```python
from build123d import *

# Parameters (mm, degrees)
F1_DEPTH = 7.62
F2_SIZE  = 2.032


with BuildPart() as f1:
    # F0 (on Top) → F1 (new body)
    with BuildSketch(Plane.XY):
        Polygon((-4.650212, 0), (0, 0), (13.123814, 0), (27.571009, 15.396307), (32.54258, 15.396307), (44.767726, 15.396307), (44.767726, 0), (58.344088, 0), (61.602417, 0), (61.602417, 13.099327), (61.602417, 15.906334), (75.450297, 0), (77.894047, 0), (92.737518, 0), (67.757033, 31.506918), (92.737518, 59.383705), (78.075059, 59.383705), (75.39035, 59.383705), (61.602417, 43.997165), (61.602417, 59.383705), (58.344088, 59.383705), (47.120962, 59.383705), align=None)
        Polygon((44.043656, 38.960008), (48.304201, 38.960008), (52.189469, 38.960008), (52.189469, 25.352303), (36.440898, 25.352303), (32.180353, 25.352303), align=None, mode=Mode.SUBTRACT)
    extrude(amount=F1_DEPTH)

    # F2
    f2_edges = [f1.edges().sort_by_distance(p)[0] for p in [
        (21.235375, 29.691853, 7.62),
        (4.236801, 0, 7.62),
        (20.347412, 7.698154, 7.62),
        (36.169368, 15.396307, 7.62),
        (44.767726, 7.698154, 7.62),
        (53.185072, 0, 7.62),
        (61.602417, 7.953167, 7.62),
        (68.526357, 7.953167, 7.62),
        (84.093908, 0, 7.62),
        (80.247276, 15.753459, 7.62),
        (80.247276, 45.445312, 7.62),
        (84.063934, 59.383705, 7.62),
        (68.496384, 51.690435, 7.62),
        (61.602417, 51.690435, 7.62),
        (54.36169, 59.383705, 7.62),
        (38.112005, 32.156156, 7.62),
        (48.116563, 38.960008, 7.62),
        (52.189469, 32.156156, 7.62),
        (42.184911, 25.352303, 7.62),
        (21.235375, 29.691853, 0),
        (4.236801, 0, 0),
        (20.347412, 7.698154, 0),
        (36.169368, 15.396307, 0),
        (44.767726, 7.698154, 0),
        (53.185072, 0, 0),
        (61.602417, 7.953167, 0),
        (68.526357, 7.953167, 0),
        (84.093908, 0, 0),
        (80.247276, 15.753459, 0),
        (80.247276, 45.445312, 0),
        (84.063934, 59.383705, 0),
        (68.496384, 51.690435, 0),
        (61.602417, 51.690435, 0),
        (54.36169, 59.383705, 0),
        (38.112005, 32.156156, 0),
        (48.116563, 38.960008, 0),
        (52.189469, 32.156156, 0),
        (42.184911, 25.352303, 0),
    ]]
    chamfer(f2_edges, length=F2_SIZE)


solid = f1.part
```
Model file for the job. Use its own axes, mm. A direction names the side the tool comes from. Coordinates: 2 decimals unless noted, no trailing zeros. Loops run counter-clockwise (first coordinate to the right, second up) from the corner with the lowest first, then second, coordinate; pieces in that order, holes last. Notation, with made-up numbers: M -11.75,37 L -7.75,37 A18 ccw -7.75,63 Z; hole C -32,43.5 d1. An arc over 180 degrees is marked long. Use CSV: the item, a comma, the result in double quotes. Start each with the question number.
1. Band-saw the part on D-D, the plane y = 53. List the corners of the cut face in (x, z).
2. Probe probe 1 along X at (y, z) = (10.5, 4.25); probe 2 along X at (y, z) = (7.5, 2.75); probe 3 along X at (y, z) = (47, 1.25). List the from-to ranges inside material, lowest first. Write a range as [from, to].
3. Flat gauge pins, fed straight in: pin 1 (1.1 mm diameter, centred on y = 7.5, z = 3.5, fed in from -X); pin 2 (1.8 mm diameter, centred on x = 36, z = 4.5, fed in from -Y); pin 3 (4 mm diameter, centred on y = 50, z = 4, fed in from +X). Where does each tip first touch, or does it go through?
4. Tool access for faces 4 (the flat face through (41.15, 24.32, 6.62)), 5 (the flat face through (60.57, 10.52, 1)), 6 (the flat face through (67.4, 10.82, 6.62)): list every direction of +Z, -Z, +X, -X, +Y, -Y with a clear straight run to the whole face (end or side of a thin tool).
5. Band-saw the part on A-A, the plane z = 4.5. List the corners of the cut face in (x, y).
6. Two-plate mould, pull along X, no slides. Class faces 1 (the flat face through (83.97, 1.03, 1)), 2 (the flat face through (20.246, 7.59, 3.785)), 3 (the flat face through (22, 29, 1)): pulls with the +X half, pulls with the -X half, needs draft (parallel to the pull), parting line crosses it, or undercut.
7. Band-saw the part on B-B, the plane y = 11.5. List the corners of the cut face in (x, z).
8. Band-saw the part on C-C, the plane x = 82.5. List the corners of the cut face in (y, z), then the cut area to 3 significant figures.
Entries:
1,outline,"M 41.56,2.03 L 44.25,0 L 59.57,0 L 61.6,2.03 L 61.6,5.59 L 59.57,7.62 L 44.25,7.62 L 41.56,5.59 Z; M 69.67,2.03 L 72.4,0 L 84.29,0 L 87.02,2.03 L 87.02,5.59 L 84.29,7.62 L 72.4,7.62 L 69.67,5.59 Z"
2,probe 1,"x = [4.5, 22.98], [44.77, 61.6], [66.31, 84.41]"
2,probe 2,"x = [1.89, 20.16], [44.77, 61.6], [68.92, 86.79]"
2,probe 3,"x = [37.36, 60.82], [65.34, 80.59]"
3,pin 1,"stops at x = 1.41"
3,pin 2,"stops at y = 15.4"
3,pin 3,"stops at x = 86.12"
4,face 4,"+Z"
4,face 5,"-Z, -Y"
4,face 6,"+Z, -Y"
5,outline,"M -4.65,0 L 13.12,0 L 27.57,15.4 L 44.77,15.4 L 44.77,0 L 61.6,0 L 61.6,15.91 L 75.45,0 L 92.74,0 L 67.76,31.51 L 92.74,59.38 L 75.39,59.38 L 61.6,44 L 61.6,59.38 L 47.12,59.38 Z; hole M 32.18,25.35 L 52.19,25.35 L 52.19,38.96 L 44.04,38.96 Z"
6,face 1,"needs draft"
6,face 2,"undercut"
6,face 3,"pulls with the -X half"
7,outline,"M 5.38,2.03 L 8.07,0 L 21.13,0 L 23.91,2.03 L 23.91,5.59 L 21.13,7.62 L 8.07,7.62 L 5.38,5.59 Z; M 44.77,2.03 L 46.8,0 L 59.57,0 L 61.6,2.03 L 61.6,5.59 L 59.57,7.62 L 46.8,7.62 L 44.77,5.59 Z; M 65.44,2.03 L 68.13,0 L 81.03,0 L 83.62,2.03 L 83.62,5.59 L 81.03,7.62 L 68.13,7.62 L 65.44,5.59 Z"
8,outline,"M 0,2.03 L 2.03,0 L 9.64,0 L 12.91,2.03 L 12.91,5.59 L 9.64,7.62 L 2.03,7.62 L 0,5.59 Z; M 47.96,2.03 L 51,0 L 57.35,0 L 59.38,2.03 L 59.38,5.59 L 57.35,7.62 L 51,7.62 L 47.96,5.59 Z"
8,area,"164 mm2"
